```python
from build123d import *

# Parameters (mm, degrees)
SKETCH1_R           = 2.5
SKETCH1_W           = 5
SKETCH1_H           = 5
BOSS_EXTRUDE1_DEPTH = 5
FILLET1_R           = 15


with BuildPart() as part:
    # Sketch1 → Boss-Extrude1 (new body)
    # profile 1 of 3: a face of its own
    with BuildSketch(Plane.XY):
        Polygon((-12.5, 8), (-12.5, -14), (-10, -14), (-5, -14), (-1.5, -14), (-1.5, -11), (-2.6, -11), (-2.6, -8.7), (-1.5, -8.7), (-1.5, -4), (1.5, -4), (1.5, -8.7), (2.6, -8.7), (2.6, -11), (1.5, -11), (1.5, -14), (5, -14), (10, -14), (12.5, -14), (12.5, 8), align=None)
        Circle(SKETCH1_R, mode=Mode.SUBTRACT)
    # profile 2 of 3: a face of its own
    with BuildSketch(Plane.XY):
        with Locations((-7.5, -16.5)):
            Rectangle(SKETCH1_W, SKETCH1_H)
    # profile 3 of 3: a face of its own
    with BuildSketch(Plane.XY):
        with Locations((7.5, -16.5)):
            Rectangle(SKETCH1_W, SKETCH1_H)
    extrude(amount=BOSS_EXTRUDE1_DEPTH)

    # Fillet1
    # the kernel refuses this fillet: 15 mm, written as the material it takes off along each edge
    with BuildSketch(Plane(origin=(-12.5, 8, -37.5), x_dir=(0, -1, 0), z_dir=(0, 0, 1)), Plane(origin=(12.5, 8, -37.5), x_dir=(-1, 0, 0), z_dir=(0, 0, 1))) as fillet1_piece_1:
        with BuildLine():
            CenterArc((FILLET1_R, FILLET1_R), FILLET1_R, 180, 90)
            Line((0, FILLET1_R), (0, 0))
            Line((0, 0), (FILLET1_R, 0))
        make_face()
    extrude(amount=80, mode=Mode.SUBTRACT)


solid = part.part
```
Check sheet for the modelled part. Datum: model origin and axes. Units: mm. A direction names the side the tool comes from. Coordinates: 2 decimals unless noted, no trailing zeros. Loops run counter-clockwise (first coordinate to the right, second up) from the corner with the lowest first, then second, coordinate; pieces in that order, holes last.
1) Sectioned sample at C-C (y = -5). Record the boundary of the cut face in (x, z).
2) Access from +Z, -Z, +X, -X, +Y, -Y to the whole of each face (thin tool, end or side, straight path). Record for faces 1 (the face through (2, -8.7, 2)), 2 (the face through (0, -4, 2)), 3 (the face through (11, -14, 2)).
3) Gauge pin test, flat ends, axial feed: pin 1 (0.6 mm diameter, centred on x = 2, z = 1.5, fed in from -Y); pin 2 (0.6 mm diameter, centred on x = -2, z = 2.5, fed in from +Y); pin 3 (1.5 mm diameter, centred on y = 3.5, z = 2.5, fed in from -X); pin 4 (12 mm diameter, centred on x = 7, y = 4.5, fed in from -Z). Record the tip position at first contact, or that the pin passes through.
4) Sectioned sample at D-D (x = 7). Record the boundary of the cut face in (y, z), and give its area (3 significant figures).
5) Sectioned sample at B-B (z = 2.15). Record the boundary of the cut face in (x, y), and give its area (3 significant figures).
6) Sectioned sample at A-A (y = -12.25). Record the boundary of the cut face in (x, z).
7) Release check for a two-part mould opening along X. For faces 4 (the face through (-2, -11, 2)), 5 (the face through (10, -17, 2)), 6 (the face through (-10, -17, 2)) record: released by +X, released by -X, zero draft, split by the parting line, or undercut.
8) Material ranges on probe 1 along X at (y, z) = (-15.25, 1.65); probe 2 along X at (y, z) = (-10.25, 1.6); probe 3 along Y at (x, z) = (0, 2.8), recorded low to high.
Check sheet entries:
1. outline: (-12.37, 0) - (-1.5, 0) - (-1.5, 5) - (-12.37, 5) - close; (1.5, 0) - (12.37, 0) - (12.37, 5) - (1.5, 5) - close
2. face 1: +Z, -Z
2. face 2: +Z, -Z, -Y
2. face 3: +Z, -Z, +X, -Y
3. pin 1: stops at y = -14
3. pin 2: stops at y = 7.4
3. pin 3: stops at x = -8.9
3. pin 4: stops at z = 0
4. outline: (-19, 0) - (4.61, 0) - (4.61, 5) - (-19, 5) - close
4. area: 118 mm2
5. outline: (-12.5, -14) - (-10, -14) - (-10, -19) - (-5, -19) - (-5, -14) - (-1.5, -14) - (-1.5, -11) - (-2.6, -11) - (-2.6, -8.7) - (-1.5, -8.7) - (-1.5, -4) - (1.5, -4) - (1.5, -8.7) - (2.6, -8.7) - (2.6, -11) - (1.5, -11) - (1.5, -14) - (5, -14) - (5, -19) - (10, -19) - (10, -14) - (12.5, -14) - (12.5, -7) arc R15 ccw to (0, 7.79) arc R15 ccw to (-12.5, -7) - close; hole circle Ø5 at (0, 0)
5. area: 449 mm2
6. outline: (-12.5, 0) - (-1.5, 0) - (-1.5, 5) - (-12.5, 5) - close; (1.5, 0) - (12.5, 0) - (12.5, 5) - (1.5, 5) - close
7. face 4: undercut
7. face 5: released by +X
7. face 6: released by -X
8. probe 1: x = -10 to -5, 5 to 10
8. probe 2: x = -12.5 to -2.6, 2.6 to 12.5
8. probe 3: y = -4 to -2.5, 2.5 to 7.79
